```python
from build123d import *

# Parameters (mm, degrees)
SKETCH1_W           = 80.01
SKETCH1_H           = 80.01
BOSS_EXTRUDE1_DEPTH = 2.54
SKETCH2_W           = 80.01
SKETCH2_H           = 80.01
SKETCH2_W_2         = 69.85
SKETCH2_H_2         = 69.85
BOSS_EXTRUDE2_DEPTH = 145.796
SKETCH3_R           = 31.75
CUT_EXTRUDE1_DEPTH  = 69.85
SKETCH5_W           = 80.01
SKETCH5_H           = 139.7
CUT_EXTRUDE3_DEPTH  = 5.08
SKETCH6_W           = 69.85
SKETCH6_H           = 69.85
SKETCH6_R           = 31.75
BOSS_EXTRUDE3_DEPTH = 145.796
CUT_EXTRUDE5_START  = -139.7
CUT_EXTRUDE5_DEPTH  = 139.7
FILLET2_R           = 25.4
SKETCH9_W           = 6.35
SKETCH9_H           = 59.944
BOSS_EXTRUDE5_DEPTH = 23
SKETCH10_R          = 2.45
SKETCH10_W          = 40.6
SKETCH10_H          = 19.9
CUT_EXTRUDE7_DEPTH  = 23
SKETCH12_W          = 14
SKETCH12_H          = 72
CUT_EXTRUDE10_DEPTH = 24.13


with BuildPart() as part:
    # Sketch1 → Boss-Extrude1 (new body)
    with BuildSketch(Plane.XY):
        Rectangle(SKETCH1_W, SKETCH1_H)
    extrude(amount=BOSS_EXTRUDE1_DEPTH)

    # Sketch2 → Boss-Extrude2 (add)
    with BuildSketch(Plane.XY.offset(2.54)):
        Rectangle(SKETCH2_W, SKETCH2_H)
        Rectangle(SKETCH2_W_2, SKETCH2_H_2, mode=Mode.SUBTRACT)
    extrude(amount=BOSS_EXTRUDE2_DEPTH)

    # Sketch3 → Cut-Extrude1 (cut)
    with BuildSketch(Plane(origin=(0, 0, 0), x_dir=(-1, 0, 0), z_dir=(0, 0, -1))):
        Circle(SKETCH3_R)
    extrude(amount=-CUT_EXTRUDE1_DEPTH, mode=Mode.SUBTRACT)

    # Sketch5 → Cut-Extrude3 (cut)
    with BuildSketch(Plane.XZ.offset(40.005)):
        with Locations((0, 78.486)):
            Rectangle(SKETCH5_W, SKETCH5_H)
    extrude(amount=-CUT_EXTRUDE3_DEPTH, mode=Mode.SUBTRACT)

    # Sketch6 → Boss-Extrude3 (add)
    with BuildSketch(Plane.XY.offset(2.54)):
        Rectangle(SKETCH6_W, SKETCH6_H)
        with Locations(Location((0, 0, 0), (0, 0, 180))):
            Circle(SKETCH6_R, mode=Mode.SUBTRACT)
    extrude(amount=BOSS_EXTRUDE3_DEPTH)

    # Sketch8 → Cut-Extrude5 (cut)
    with BuildSketch(Plane.XY.offset(148.336).offset(CUT_EXTRUDE5_START)):
        with BuildLine():
            ThreePointArc((31.75, 0), (0, -31.75), (-31.75, 0))
            Line((-31.75, 0), (-31.75, -34.925))
            Line((-31.75, -34.925), (31.75, -34.925))
            Line((31.75, -34.925), (31.75, 0))
        make_face()
    extrude(amount=CUT_EXTRUDE5_DEPTH, mode=Mode.SUBTRACT)

    # Fillet2
    # the kernel refuses this fillet: 25.4 mm, written as the material it takes off along each edge
    with BuildSketch(Plane(origin=(31.75, -34.925, 8.636), x_dir=(1, 0, 0), z_dir=(0, 0, 1))) as fillet2_piece_1:
        with BuildLine():
            CenterArc((25.4, 18.740570295), FILLET2_R, 180, 47.545849796)
            Line((0, 18.740570295), (0, 0))
            Line((0, 0), (8.255, 0))
        make_face()
    extrude(amount=186.551425739, mode=Mode.SUBTRACT)
    with BuildSketch(Plane(origin=(-31.75, -34.925, 8.636), x_dir=(0, 1, 0), z_dir=(0, 0, 1))) as fillet2_piece_2:
        with BuildLine():
            CenterArc((18.740570295, 25.4), FILLET2_R, 222.454150204, 47.545849796)
            Line((0, 8.255), (0, 0))
            Line((0, 0), (18.740570295, 0))
        make_face()
    extrude(amount=186.551425739, mode=Mode.SUBTRACT)

    # Sketch9 → Boss-Extrude5 (add)
    with BuildSketch(Plane(origin=(0, 40.005, 0), x_dir=(1, 0, 0), z_dir=(0, 1, 0))):
        with Locations((20.193, -42.418)):
            Rectangle(SKETCH9_W, SKETCH9_H)
    extrude(amount=BOSS_EXTRUDE5_DEPTH)

    # Sketch10 → Cut-Extrude7 (cut)
    with BuildSketch(Plane(origin=(23.368, 0, 0), x_dir=(0, 0, -1), z_dir=(1, 0, 0))):
        with Locations((-69.659214709, 44.502596375)):
            Circle(SKETCH10_R)
        with Locations((-69.659214709, 56.402596375)):
            Circle(SKETCH10_R)
        with Locations((-18.639214709, 44.502596375)):
            Circle(SKETCH10_R)
        with Locations((-18.639214709, 56.244452771)):
            Circle(SKETCH10_R)
        with Locations((-44.149214709, 50.452596375)):
            Rectangle(SKETCH10_W, SKETCH10_H)
    extrude(amount=-CUT_EXTRUDE7_DEPTH, mode=Mode.SUBTRACT)

    # Sketch12 → Cut-Extrude10 (cut)
    with BuildSketch(Plane(origin=(0, 40.005, 0), x_dir=(1, 0, 0), z_dir=(0, 1, 0))):
        with Locations((1.568, -35.570235268)):
            Rectangle(SKETCH12_W, SKETCH12_H)
    extrude(amount=-CUT_EXTRUDE10_DEPTH, mode=Mode.SUBTRACT)


solid = part.part
```
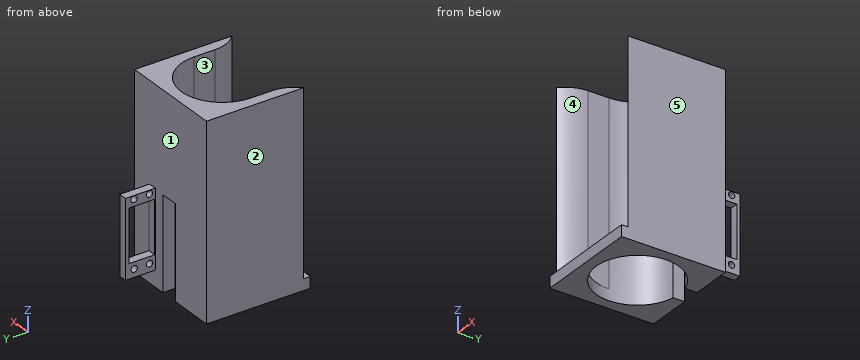
Build history of the part. All positions in model axes, mm. Face numbers are marked on the shaded views. A direction names the side the tool comes from. Round coordinates to 2 decimals unless told otherwise and drop trailing zeros. Loops run counter-clockwise (first coordinate to the right, second up) from the corner with the lowest first, then second, coordinate; pieces in that order, holes last.
Item 1: Drill centre lines: line 1 along X through (y, z) = (0, 86) (3 decimals); line 2 along X through (y, z) = (32.5, 56.5) (3 decimals); line 3 along Z through (x, y) = (-24, -30). Where is each one in solid material? Low to high.
Item 2: Which spindle directions (+Z, -Z, +X, -X, +Y, -Y) get a long thin tool onto all of the face, cutting with end or side? Do the marked faces 4 and 5. Say none if no direction does.
Item 3: Two-plate mould, pull along X, no slides. Class the marked faces 1, 2 and 3: released by +X, released by -X, zero draft, split by the parting line, or undercut.
Item 4: Saw through at A-A (x = 0). List the corners of the cut face in (y, z) (3 decimals).
Item 5: Saw through at C-C (z = 19.5). List the corners of the cut face in (x, y) (3 decimals), then the cut area to 3 significant figures.
Item 6: Saw through at B-B (y = -12.5). List the corners of the cut face in (x, z) (3 decimals), then the cut area to 3 significant figures.
Item 7: Pin check, flat tips, straight feed: P1, Ø5, axis at x = -25.5, z = 78, coming from the -Y side; P2, Ø3, axis at x = -31, z = 118, coming from the +Y side (3 decimals); P3, Ø8, axis at y = 56.24, z = 18.64, coming from the +X side. Stop position of each tip, or through.
Item 8: Saw through at D-D (x = 21). List the corners of the cut face in (y, z) (3 decimals).
Worked answers:
1. line 1: x = -40.005 to -31.75, 31.75 to 40.005
1. line 2: x = -40.005 to -5.432, 8.568 to 40.005
1. line 3: z = 0 to 8.64
2. face 4: +Z, -Y
2. face 5: +Z, -Z, +X, +Y, -Y
3. face 1: zero draft
3. face 2: released by -X
3. face 3: undercut
4. outline: (-40.005, 0) - (-31.75, 0) - (-31.75, 8.636) - (-40.005, 8.636) - close; (31.75, 71.57) - (40.005, 71.57) - (40.005, 148.336) - (31.75, 148.336) - close
5. outline: (-40.005, -34.925) arc R25.4 ccw to (-31.75, -16.184) - (-31.75, 0) arc R31.75 cw to (-5.432, 31.282) - (-5.432, 40.005) - (-40.005, 40.005) - close; (8.568, 30.572) arc R31.75 cw to (31.75, 0) - (31.75, -16.184) arc R25.4 ccw to (40.005, -34.925) - (40.005, 40.005) - (23.368, 40.005) - (23.368, 42.209) - (17.018, 42.209) - (17.018, 40.005) - (8.568, 40.005) - close; (17.018, 46.796) - (23.368, 46.796) - (23.368, 53.951) - (17.018, 53.951) - close; (17.018, 58.538) - (23.368, 58.538) - (23.368, 63.005) - (17.018, 63.005) - close
5. area: 2,070 mm2
6. outline: (-40.005, 0) - (-29.186, 0) - (-29.186, 8.636) - (-31.75, 8.636) - (-31.75, 148.336) - (-40.005, 148.336) - close; (29.186, 0) - (40.005, 0) - (40.005, 148.336) - (31.75, 148.336) - (31.75, 8.636) - (29.186, 8.636) - close
6. area: 2,490 mm2
7. P1: stops at y = 14.97
7. P2: stops at y = 40.005
7. P3: stops at x = 23.37
8. outline: (-40.005, 0) - (-23.813, 0) - (-23.813, 8.636) - (-40.005, 8.636) - close; (23.813, 0) - (40.005, 0) - (40.005, 12.446) - (63.005, 12.446) - (63.005, 72.39) - (40.005, 72.39) - (40.005, 148.336) - (23.813, 148.336) - close; hole (40.503, 23.849) - (60.403, 23.849) - (60.403, 64.449) - (40.503, 64.449) - close; hole circle Ø4.9 at (44.503, 18.639); hole circle Ø4.9 at (44.503, 69.659); hole circle Ø4.9 at (56.244, 18.639); hole circle Ø4.9 at (56.403, 69.659)
